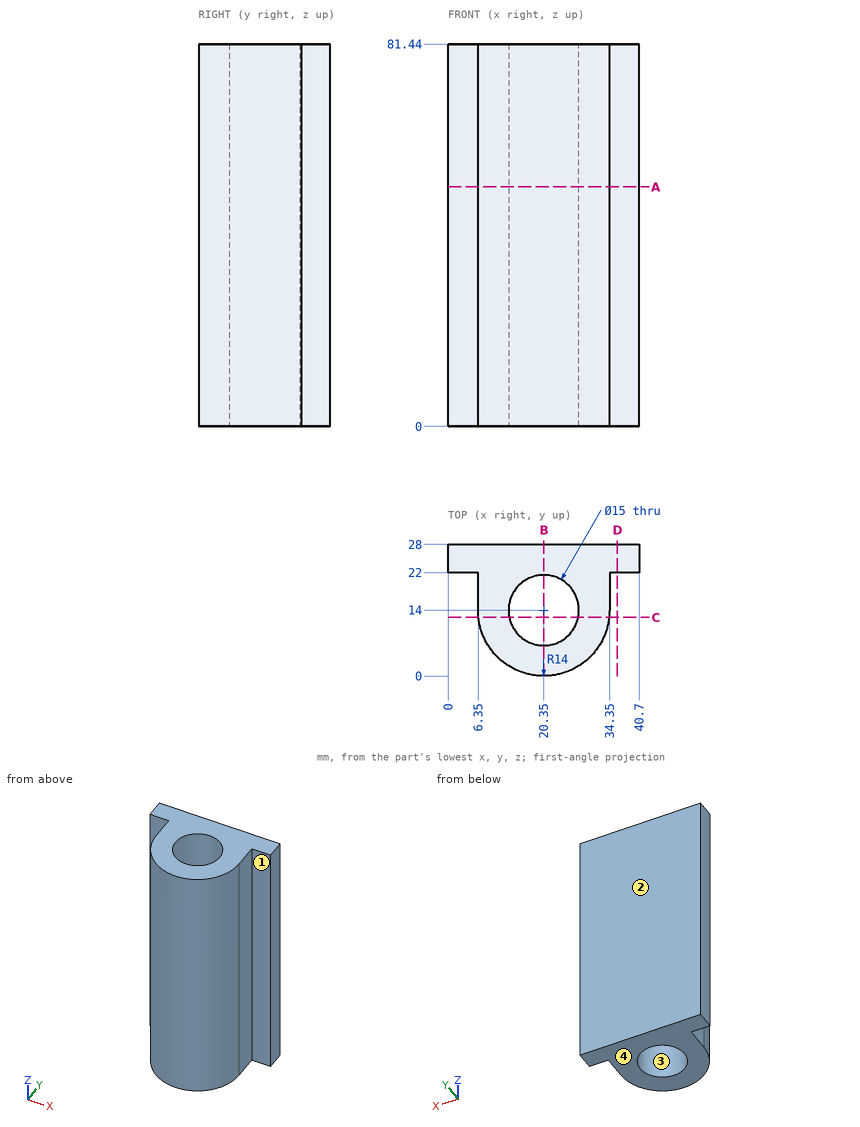
Print and shaded views of the part. All mm, measured from the part's lowest x, y and z. Coordinates: 2 decimals unless noted, no trailing zeros. Order: outer loops, then holes, each group sorted by start corner. A loop starts at its lowest first (then second) coordinate and runs counter-clockwise, first axis right, second up. Notation, with made-up numbers: (14.5, 54) - (36.5, 54) arc R7 ccw to (36.5, 66) - close; hole circle Ø10 at (17.25, 21.5). An arc over 180 degrees is marked (long way). Return JSON: item names as keys, results as strings. Group by question number.
Item 1: Pin check, flat tips, straight feed: pin 1 (4 mm diameter, centred on y = 10.5, z = 72, fed in from -X); pin 2 (1 mm diameter, centred on y = 20.5, z = 49, fed in from +X); pin 3 (4 mm diameter, centred on y = 7.5, z = 47, fed in from -X); pin 4 (4 mm diameter, centred on x = 22.5, z = 34, fed in from -Y). Stop position of each tip, or through.
Item 2: Pull direction Y, two halves, no side cores. Call the marked faces 1, 2, 3 and 4: pulls with the +Y half, pulls with the -Y half, needs draft (parallel to the pull), parting line crosses it, or undercut.
Item 3: Cut at B-B (x = 20.35). List the corners of the cut face in (y, z).
Item 4: Cut at C-C (y = 12.5). List the corners of the cut face in (x, z).
Item 5: Cut at D-D (x = 36). List the corners of the cut face in (y, z).
Item 6: Drill centre lines: probe 1 along Y at (x, z) = (20, 34); probe 2 along X at (y, z) = (11.75, 28); probe 3 along X at (y, z) = (12.5, 13). Where is each one in solid material? Low to high. Write a range as from..to.
Item 7: Cut at A-A (z = 51). List the corners of the cut face in (x, y).
Check values:
{
 "1": {"pin 1": "stops at x = 6.43", "pin 2": "stops at x = 34.35", "pin 3": "stops at x = 7.09", "pin 4": "stops at y = 0"},
 "2": {"face 1": "pulls with the -Y half", "face 2": "pulls with the +Y half", "face 3": "undercut", "face 4": "needs draft"},
 "3": {"outline": "(0, 0) - (6.5, 0) - (6.5, 81.44) - (0, 81.44) - close; (21.5, 0) - (28, 0) - (28, 81.44) - (21.5, 81.44) - close"},
 "4": {"outline": "(6.43, 0) - (13, 0) - (13, 81.44) - (6.43, 81.44) - close; (27.7, 0) - (34.27, 0) - (34.27, 81.44) - (27.7, 81.44) - close"},
 "5": {"outline": "(22, 0) - (28, 0) - (28, 81.44) - (22, 81.44) - close"},
 "6": {"probe 1": "y = 0..6.51, 21.49..28", "probe 2": "x = 6.53..13.2, 27.5..34.17", "probe 3": "x = 6.43..13, 27.7..34.27"},
 "7": {"outline": "(0, 22) - (6.35, 22) - (6.35, 14) arc R14 ccw to (34.35, 14) - (34.35, 22) - (40.7, 22) - (40.7, 28) - (0, 28) - close; hole circle Ø15 at (20.35, 14)"}
}
